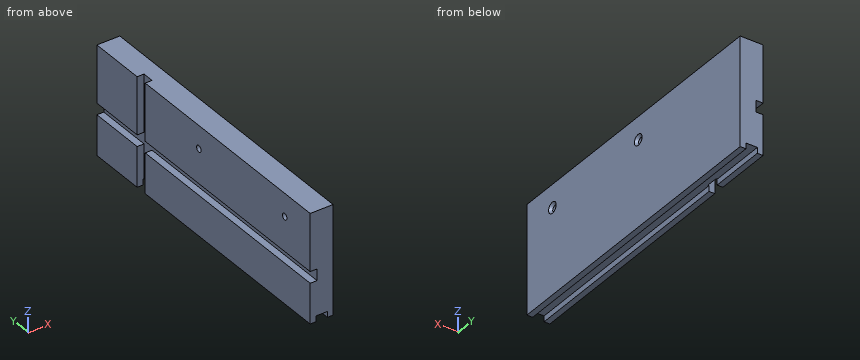
Autodesk Inventor part; units mm, degrees
ref_plane "YZ Plane" through (0, 0, 0) normal (1, 0, 0) x (0, 1, 0)
ref_plane "XZ Plane" through (0, 0, 0) normal (0, 1, 0) x (-1, 0, 0)
ref_plane "XY Plane" through (0, 0, 0) normal (0, 0, 1) x (1, 0, 0)
sketch "Sketch1" plane through (0, 0, 0) normal (1, 0, 0) x (0, 1, 0)
  line L0 (-57.15, 57.15) -> (57.15, 57.15)
  line L1 (57.15, 57.15) -> (57.15, 0)
  line L2 (57.15, 0) -> (-57.15, 0)
  line L3 (-57.15, 0) -> (-57.15, 57.15)
  line L4 (-57.15, 57.15) -> (57.15, 0) construction
  line L5 (57.15, 57.15) -> (-57.15, 0) construction
  line L6 (-26.9875, 0) -> (26.9875, 0)
  line L7 (26.9875, 0) -> (26.9875, 26.9875)
  line L8 (26.9875, 26.9875) -> (-26.9875, 26.9875)
  line L9 (-26.9875, 26.9875) -> (-26.9875, 0)
  line L10 (-26.9875, 26.9875) -> (-26.9875, 57.15)
  line L11 (26.9875, 26.9875) -> (57.15, 26.9875)
  point P0 (0, 0)
  point P1 (0, 28.575)
  point P2 (0, 0)
  dimension "d5" = 114.3
  dimension "d6" = 57.15
  dimension "d7" = 53.975
  dimension "d8" = 26.9875
extrude "Extrusion1" add sketch "Sketch1" along normal blind 6.35 contours L0 L1 L11 L8 L10
sketch "Sketch2" plane through (0, -26.9875, 26.9875) normal (0, 0, -1) x (-1, 0, 0)
  line L0 (0, 0) -> (0, 84.1375)
  line L1 (0, 84.1375) -> (-6.35, 84.1375)
  line L2 (-6.35, 0) -> (-6.35, 84.1375)
  line L3 (0, 0) -> (-6.35, 0)
  line L4 (-3.175, 0) -> (-3.175, 84.1375)
  line L5 (-4.7625, 0) -> (-1.5875, 0)
  line L6 (-1.5875, 0) -> (-1.5875, 84.1375)
  line L7 (-1.5875, 84.1375) -> (-4.7625, 84.1375)
  line L8 (-4.7625, 84.1375) -> (-4.7625, 0)
  line L9 (-4.7625, 0) -> (-1.5875, 84.1375) construction
  line L10 (-1.5875, 0) -> (-4.7625, 84.1375) construction
  point P0 (0, 26.9875)
  point P1 (-3.175, 42.0688)
  dimension "d11" = 3.175
extrude "Extrusion2" cut sketch "Sketch2" against normal blind 1.5875 contours L3 L4 L1 L6 | L3 L8 L1 L4
sketch "Sketch3" plane through (6.35, 0, 0) normal (1, 0, 0) x (0, 0, -1)
  line L0 (-26.9875, -26.9875) -> (-26.9875, 57.15)
  line L1 (-26.9875, 57.15) -> (-57.15, 57.15)
  line L2 (-57.15, 57.15) -> (-57.15, -26.9875)
  line L3 (-57.15, -26.9875) -> (-26.9875, -26.9875)
  line L4 (-50.8, -16.9333) -> (-50.8, 16.9333)
  point P0 (0, 0)
  dimension "d16" = 40.2167
  dimension "d31" = 33.8667
  dimension "d32" = 6.35
hole "Hole1" at (6.35, -16.9333, 50.8) at (6.35, 16.9333, 50.8) direction (-1, 0, 0) diameter 1.778 end through all countersink diameter 3.023 countersink angle 82
sketch "Sketch4" plane through (0, 0, 0) normal (-1, 0, 0) x (0, 0, 1)
  line L0 (-38.1, -38.1) -> (38.1, -38.1)
  line L1 (38.1, -38.1) -> (38.1, 38.1)
  line L2 (38.1, 38.1) -> (-38.1, 38.1)
  line L3 (-38.1, 38.1) -> (-38.1, -38.1)
  line L4 (-38.1, -38.1) -> (38.1, 38.1) construction
  line L5 (38.1, -38.1) -> (-38.1, 38.1) construction
  line L6 (-41.275, 41.275) -> (41.275, 41.275)
  line L7 (41.275, 41.275) -> (41.275, -41.275)
  line L8 (41.275, -41.275) -> (-41.275, -41.275)
  line L9 (-41.275, -41.275) -> (-41.275, 41.275)
  line L10 (-41.275, 41.275) -> (41.275, -41.275) construction
  line L11 (41.275, 41.275) -> (-41.275, -41.275) construction
  line L12 (26.9875, 57.15) -> (57.15, 57.15)
  line L13 (38.1, 38.1) -> (41.275, 38.1)
  line L14 (41.275, 38.1) -> (41.275, 57.15)
  line L15 (41.275, 57.15) -> (38.1, 57.15)
  line L16 (38.1, 57.15) -> (38.1, 38.1)
  line L17 (38.1, 38.1) -> (57.15, 38.1)
  line L18 (57.15, 38.1) -> (57.15, 41.275)
  line L19 (57.15, 41.275) -> (38.1, 41.275)
  line L20 (38.1, 41.275) -> (38.1, 38.1)
  line L21 (57.15, 57.15) -> (57.15, -26.9875)
  point P0 (0, 0)
  dimension "d24" = 76.2
  dimension "d25" = 76.2
  dimension "d26" = 3.175
  dimension "d27" = 3.175
extrude "Extrusion3" cut sketch "Sketch4" against normal blind 1.905 contours L13 L7 L8 L9 L6 L16 | L16 L6 L7 L13 | L7 L19 L18 L17 | L16 L12 L14 L6
equation "\"d5\" = width + 2 * acrylicThickness"
equation "\"d6\" = acrylicThickness + 0.5 * height"
equation "\"d7\" = sensorHolderSensorWidth"
equation "\"d8\" = 0.5 * sensorHolderSesnorHeight"
equation "\"d9\" = acrylicThickness"
equation "\"d11\" = oRingWidth"
equation "\"d12\" = 0.5 * oRingWidth"
equation "\"d16\" = 0.333333 * width + acrylicThickness"
equation "\"d31\" = 0.333333 * width"
equation "\"d32\" = acrylicThickness"
equation "\"d24\" = 0.25 * sensorHolderFlushORingID"
equation "\"d25\" = 0.25 * sensorHolderFlushORingID"
equation "\"d26\" = oRingWidth"
equation "\"d27\" = oRingWidth"
equation "\"acrylicThickness\" = 6.35"
equation "\"height\" = 101.6"
equation "\"width\" = 101.6"
equation "\"depth\" = 101.6"
equation "\"mirrorAngle\" = 5deg"
equation "\"detectorWidth\" = 52"
equation "\"detectorHeight\" = 52"
equation "\"mirrorThickness\" = 3"
equation "\"fresnelThickness\" = 0.1"
equation "\"focalLength\" = 76.2"
equation "\"ior\" = 1.49"
equation "\"centerThickness\" = 1.524"
equation "\"fresnelAngle\" = 90deg"
equation "\"fresnelEffectiveDiameter\" = 76.2"
equation "\"mirrorSuppourtWidth\" = 38.1"
equation "\"backGrooveBit\" = 4.8006"
equation "\"sensorHolderWidth\" = 88.9"
equation "\"sensorHolderHeight\" = 88.9"
equation "\"sensorHolderSesnorHeight\" = 53.975"
equation "\"sensorHolderSensorWidth\" = 53.975"
equation "\"sensorHolderSensorHeight\" = 53.975"
equation "\"sensorHolderORingGroove\" = 3.175"
equation "\"sensorHolderORing\" = 3.175"
equation "\"sensorHolderFlushORing\" = 3.175"
equation "\"sensorHolderFlushORingID\" = 304.8"
equation "\"frontBackORingID\" = 419.1"
equation "\"oRingWidth\" = 3.175"
equation "\"sensorHolderORingID\" = 203.2"
equation "\"topBottomHorizontalMirrorGroove\" = 12.7"
equation "\"backMirrorGroove\" = 6.35"
equation "\"mirrorGroove\" = 19.05"
equation "\"fresnelChamfer\" = 6.35"
equation "\"mirrorGrooveFillet\" = 6.35"
equation "\"mirrorGrooveDrill\" = 6.35"
equation "\"mirrorGrooveMill\" = 3.175"
equation "\"fresnelMirrorChamfer\" = 6.35"
equation "\"detectorOpeningWidth\" = 76.2"
equation "\"detectorOpeningHeight\" = 76.2"
properties part number "sensorHolder" material "ABS Plastic"
CAD build for the part. Positions are in the model's coordinates, mm. Give positions to 0.01 mm unless a question says otherwise; leave off trailing zeros. Write each question's results on one line, items separated by ' | '.
1. Probe L1, parallel to Y at x = 2, z = 50.8; L2, parallel to Y at x = 6.25, z = 51.5; L3, parallel to Z at x = 1.75, y = 16.5 (3 decimals). List the from-to ranges inside material, lowest first. Write a range as from..to.
Calculated:
L1: y = -26.99..-17.82, -16.04..16.04, 17.82..57.15 | L2: y = -26.99..-18.17, -15.69..15.69, 18.17..57.15 | L3: z = 28.575..38.1, 41.275..50.024, 51.576..57.15
2. Pin check, flat tips, straight feed: pin 1 (8 mm diameter, centred on y = 9, z = 51.5, fed in from -X); pin 2 (1.6 mm diameter, centred on x = 2.5, y = -1.5, fed in from -Z) (3 decimals). Stop position of each tip, or through.
Calculated:
pin 1: stops at x = 0 | pin 2: stops at z = 28.575
3. Saw through at A-A on z = 50.8. Count the separate pieces of the cut face and the enclosed holes in it, and give its area (3 significant figures).
Calculated:
separate pieces: 3 | enclosed holes: 0 | area: 505 mm2
